from build123d import *

# Parameters (mm, degrees)
SKETCH1_W               = 75
SKETCH1_H               = 50
BOSS_EXTRUDE1_DEPTH     = 10
BOSS_EXTRUDE2_DEPTH     = 10
FILLET1_R               = 10
SKETCH4_R               = 5
CUT_EXTRUDE1_DEPTH      = 11
FILLET1_OF_MIRROR1_R    = 10
SKETCH5_R               = 2.5
CUT_EXTRUDE2_DEPTH      = 11
MIRROR3_COPY_1_SKETCH_R = 2.5
MIRROR3_COPY_1_DEPTH    = 11
SKETCH6_W               = 30
SKETCH6_H               = 30
CUT_EXTRUDE3_DEPTH      = 5
FILLET2_R               = 2


with BuildPart() as part:
    # Sketch1 → Boss-Extrude1 (new body)
    with BuildSketch(Plane(origin=(0, 0, 0), x_dir=(1, 0, 0), z_dir=(0, 1, 0))):
        with Locations((37.5, 25)):
            Rectangle(SKETCH1_W, SKETCH1_H)
    extrude(amount=BOSS_EXTRUDE1_DEPTH)

    # Sketch2 → Boss-Extrude2 (add)
    with BuildSketch(Plane.XY):
        with BuildLine():
            Line((52.5, 20), (57.5, 10))
            Line((57.5, 10), (17.5, 10))
            Line((17.5, 10), (22.5, 20))
            ThreePointArc((22.5, 20), (37.5, 35), (52.5, 20))
        make_face()
    boss_extrude2 = extrude(amount=-BOSS_EXTRUDE2_DEPTH)

    # Fillet1
    fillet1_edges = [part.edges().sort_by_distance(p)[0] for p in [
        (22.5, 20, -5),
        (52.5, 20, -5),
        (57.5, 10, -5),
        (17.5, 10, -5),
    ]]
    fillet(fillet1_edges, radius=FILLET1_R)

    # Sketch4 → Cut-Extrude1 (cut, through all)
    with BuildSketch(Plane(origin=(0, 0, -10), x_dir=(-1, 0, 0), z_dir=(0, 0, -1))):
        with Locations((-37.5, 20)):
            Circle(SKETCH4_R)
    cut_extrude1 = extrude(amount=-CUT_EXTRUDE1_DEPTH, mode=Mode.SUBTRACT)

    # Mirror1: Boss-Extrude2, Cut-Extrude1 across plane
    add(boss_extrude2.mirror(Plane(origin=(0, 0, -25), x_dir=(1, 0, 0), z_dir=(0, 0, -1))))
    add(cut_extrude1.mirror(Plane(origin=(0, 0, -25), x_dir=(1, 0, 0), z_dir=(0, 0, -1))), mode=Mode.SUBTRACT)

    # Fillet1 of Mirror1
    fillet1_of_mirror1_edges = [part.edges().sort_by_distance(p)[0] for p in [
        (22.5, 20, -45),
        (52.5, 20, -45),
        (57.5, 10, -45),
        (17.5, 10, -45),
    ]]
    fillet(fillet1_of_mirror1_edges, radius=FILLET1_OF_MIRROR1_R)

    # Sketch5 → Cut-Extrude2 (cut, through all)
    with BuildSketch(Plane(origin=(0, 10, 0), x_dir=(1, 0, 0), z_dir=(0, 1, 0))):
        with Locations((5, 5)):
            Circle(SKETCH5_R)
    cut_extrude2 = extrude(amount=-CUT_EXTRUDE2_DEPTH, mode=Mode.SUBTRACT)

    # Mirror2: Cut-Extrude2 across plane
    add(cut_extrude2.mirror(Plane(origin=(0, 0, -25), x_dir=(1, 0, 0), z_dir=(0, 0, -1))), mode=Mode.SUBTRACT)

    # Mirror3: Cut-Extrude2 across plane
    add(cut_extrude2.mirror(Plane(origin=(37.5, 0, 0), x_dir=(0, 0, 1), z_dir=(1, 0, 0))), mode=Mode.SUBTRACT)

    # Mirror3 copy 1 sketch → Mirror3 copy 1 (cut, through all)
    with BuildSketch(Plane(origin=(75, 10, -50), x_dir=(-1, 0, 0), z_dir=(0, 1, 0))):
        with Locations((5, 5)):
            Circle(MIRROR3_COPY_1_SKETCH_R)
    extrude(amount=-MIRROR3_COPY_1_DEPTH, mode=Mode.SUBTRACT)

    # Sketch6 → Cut-Extrude3 (cut)
    with BuildSketch(Plane(origin=(0, 10, 0), x_dir=(1, 0, 0), z_dir=(0, 1, 0))):
        with Locations((37.5, 25)):
            Rectangle(SKETCH6_W, SKETCH6_H)
    extrude(amount=-CUT_EXTRUDE3_DEPTH, mode=Mode.SUBTRACT)

    # Fillet2
    fillet2_edges = [part.edges().sort_by_distance(p)[0] for p in [
        (22.5, 7.5, -10),
        (22.5, 7.5, -40),
        (52.5, 7.5, -40),
        (52.5, 7.5, -10),
    ]]
    fillet(fillet2_edges, radius=FILLET2_R)


solid = part.part
Part model, mm, in its own coordinate system. A direction names the side the tool comes from. Round coordinates to 2 decimals unless told otherwise and drop trailing zeros. Order: outer loops, then holes, each group sorted by start corner. A loop starts at its lowest first (then second) coordinate and runs counter-clockwise, first axis right, second up. Notation, with made-up numbers: (6, 7.25) -> (65, 7.25) arc R19 ccw to (65, 32.25) -> close; hole circle Ø3 at (-22.75, -22.75). An arc over 180 degrees is marked (long way). Put each result on its own line as item: value.
Q1. Tool access for faces 4 (the face through (51.9, 7.46, -10.57)), 5 (the face through (37.192, 34.997, -45.07)), 6 (the face through (65, 10, -25)), 7 (the face through (9, 10, -25)), 8 (the face through (41.5, 17, -44.9)): list every direction of +Z, -Z, +X, -X, +Y, -Y with a clear straight run to the whole face (end or side of a thin tool).
From the geometry:
face 4: +Y
face 5: +Z, -Z, +Y
face 6: +X, +Y
face 7: -X, +Y
face 8: +Z, -Z
Q2. Band-saw the part on C-C (y = 8.5). Give the cut face in (x, z), and give its area (3 significant figures).
From the geometry:
outline: (0, -50) -> (75, -50) -> (75, 0) -> (0, 0) -> close; hole circle Ø5 at (5, -45); hole circle Ø5 at (5, -5); hole (22.5, -38) arc R2 ccw to (24.5, -40) -> (50.5, -40) arc R2 ccw to (52.5, -38) -> (52.5, -12) arc R2 ccw to (50.5, -10) -> (24.5, -10) arc R2 ccw to (22.5, -12) -> close; hole circle Ø5 at (70, -45); hole circle Ø5 at (70, -5)
area: 2,770 mm2
Q3. Band-saw the part on D-D (y = 28). Give the cut face in (x, z).
From the geometry:
outline: (24.81, -50) -> (50.19, -50) -> (50.19, -40) -> (24.81, -40) -> close; (24.81, -10) -> (50.19, -10) -> (50.19, 0) -> (24.81, 0) -> close
Q4. Wall check: line 1 (X direction, y = 2.75, z = -5); line 2 (Z direction, x = 70, y = 5); line 3 (Z direction, x = 34, y = 24). Give the ranges that are in metal, low to high. Write a range as [from, to].
From the geometry:
line 1: x = [0, 2.5], [7.5, 67.5], [72.5, 75]
line 2: z = [-50, -47.5], [-42.5, -7.5], [-2.5, 0]
line 3: z = [-50, -40], [-10, 0]
Q5. Band-saw the part on B-B (z = -45). Give the cut face in (x, y).
From the geometry:
outline: (0, 0) -> (2.5, 0) -> (2.5, 10) -> (0, 10) -> close; (7.5, 0) -> (67.5, 0) -> (67.5, 10) -> (63.68, 10) arc R10 cw to (54.74, 15.53) -> (53.42, 18.17) arc R10 cw to (52.42, 21.58) arc R15 ccw to (22.58, 21.58) arc R10 cw to (21.58, 18.17) -> (20.26, 15.53) arc R10 cw to (11.32, 10) -> (7.5, 10) -> close; (72.5, 0) -> (75, 0) -> (75, 10) -> (72.5, 10) -> close; hole circle Ø10 at (37.5, 20)
Q6. Band-saw the part on A-A (x = 70). Give the cut face in (y, z), and give its area (3 significant figures).
From the geometry:
outline: (0, -50) -> (10, -50) -> (10, -47.5) -> (0, -47.5) -> close; (0, -42.5) -> (10, -42.5) -> (10, -7.5) -> (0, -7.5) -> close; (0, -2.5) -> (10, -2.5) -> (10, 0) -> (0, 0) -> close
area: 400 mm2
Q7. Pin check, flat tips, straight feed: pin 1 Ø4.5 at (x, z) = (70, -45) entering from -Y; pin 2 Ø7.5 at (x, z) = (57, -29.5) entering from +Y; pin 3 Ø8 at (y, z) = (31, -10) entering from -X; pin 4 Ø12 at (x, z) = (29, -31.5) entering from +Y. Stop position of each tip, or through.
From the geometry:
pin 1: passes through
pin 2: stops at y = 10
pin 3: stops at x = 24.23
pin 4: stops at y = 5
Q8. Pull direction Z, two halves, no side cores. Call faces 1 (the face through (7.385, 5.07, -5.751)), 2 (the face through (37, 13, 0)), 3 (the face through (21, 17, -5)): pulls with the +Z half, pulls with the -Z half, needs draft (parallel to the pull), parting line crosses it, or undercut.
From the geometry:
face 1: undercut
face 2: pulls with the +Z half
face 3: needs draft
